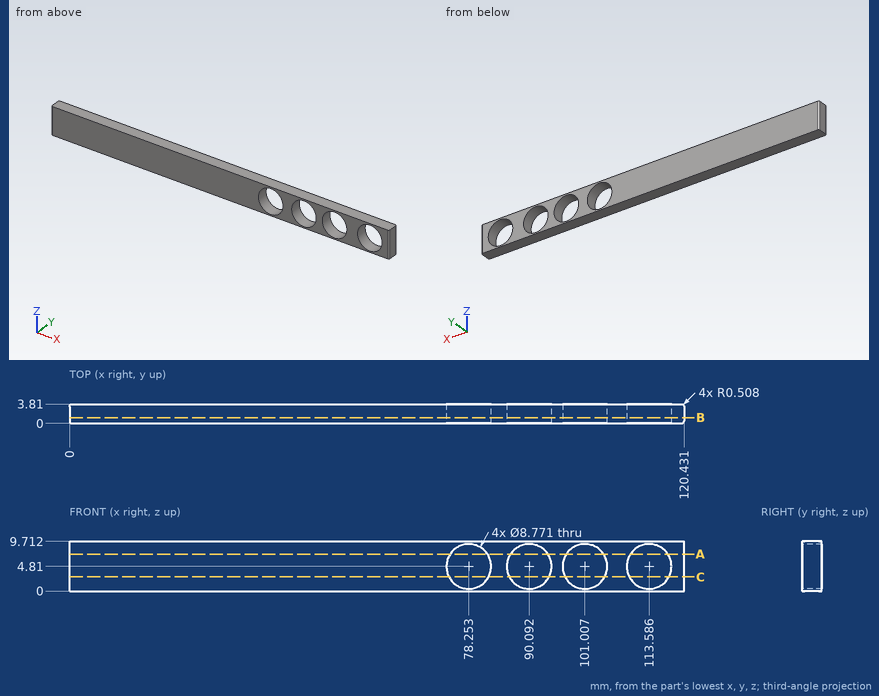
Study the drawing (mm; zero at the part's minimum x, y, z) and answer. Coordinates: 2 decimals unless noted, no trailing zeros. Order: outer loops, then holes, each group sorted by start corner. A loop starts at its lowest first (then second) coordinate and runs counter-clockwise, first axis right, second up. Notation, with made-up numbers: M 62.25,77 L 101.25,77 A33 cw 101.25,112 Z; hole C 42.5,-5.75 d4. An arc over 180 degrees is marked long. Answer as a JSON object with one key per item and string values. Group by question number.
1. Section B-B on y = 1.15 is taken. Write down the section's boundary in (x, z) (1 decimal).
2. Section C-C on z = 2.75 is taken. Write down the section's boundary in (x, y) (1 decimal).
3. Straight lines are drawn through the part: line 1 (X direction, y = 2.85, z = 4.5); line 2 (X direction, y = 1.7, z = 4); line 3 (Z direction, x = 92, y = 2.6). For each, find the intervals that lie inside material, in ascending order.
4. Section A-A on z = 7.25 is taken. Write down the section's boundary in (x, y).
Values follow:
{
 "1": {"outline": "M 0,0 L 120.4,0 L 120.4,9.7 L 0,9.7 Z; hole C 78.3,4.8 d8.8; hole C 90.1,4.8 d8.8; hole C 101,4.8 d8.8; hole C 113.6,4.8 d8.8"},
 "2": {"outline": "M 0,0.5 A0.5 ccw 0.5,0 L 74.4,0 L 74.4,3.8 L 0.5,3.8 A0.5 ccw 0,3.3 Z; M 82.1,0 L 86.2,0 L 86.2,3.8 L 82.1,3.8 Z; M 94,0 L 97.1,0 L 97.1,3.8 L 94,3.8 Z; M 104.9,0 L 109.7,0 L 109.7,3.8 L 104.9,3.8 Z; M 117.5,0 L 119.9,0 A0.5 ccw 120.4,0.5 L 120.4,3.3 A0.5 ccw 119.9,3.8 L 117.5,3.8 Z"},
 "3": {"line 1": "0 to 73.88, 82.63 to 85.72, 94.47 to 96.63, 105.38 to 109.21, 117.96 to 120.43", "line 2": "0 to 73.94, 82.56 to 85.78, 94.4 to 96.7, 105.32 to 109.28, 117.9 to 120.43", "line 3": "0 to 0.86, 8.76 to 9.71"},
 "4": {"outline": "M 0,0.51 A0.51 ccw 0.51,0 L 74.61,0 L 74.61,3.81 L 0.51,3.81 A0.51 ccw 0,3.3 Z; M 81.9,0 L 86.45,0 L 86.45,3.81 L 81.9,3.81 Z; M 93.74,0 L 97.36,0 L 97.36,3.81 L 93.74,3.81 Z; M 104.65,0 L 109.94,0 L 109.94,3.81 L 104.65,3.81 Z; M 117.23,0 L 119.92,0 A0.51 ccw 120.43,0.51 L 120.43,3.3 A0.51 ccw 119.92,3.81 L 117.23,3.81 Z"}
}
